Input: part model. Units: mm. Frame: model coordinates. Face numbers are marked on the shaded views. A direction names the side the tool comes from. Give positions to 0.01 mm unless a question says otherwise; leave off trailing zeros. Write each loop counter-clockwise with the first axis right and the second up, starting at its lowest first coordinate (ties: lowest second). Pieces come first, ordered by that corner, then holes. Notation, with made-up numbers: (-36, -17) -> (-12, -17) arc R19 cw to (-12, -2) -> close; hole circle Ø3 at (37.25, 26.25). An arc over 180 degrees is marked (long way). Answer as a JSON object with one key per item and string values. Group by question number.
from build123d import *

# Parameters (mm, degrees)
BOSS_EXTRUDE1_DEPTH       = 0.5
BOSS_EXTRUDE1_DEPTH_BACK  = 1
SKETCH1_R                 = 25
SKETCH17_R                = 24
SKETCH17_R_2              = 23
BOSS_EXTRUDE15_DEPTH      = 2
SKETCH2_R                 = 1
BOSS_EXTRUDE2_DEPTH       = 10
SKETCH12_W                = 23.219340148
SKETCH12_H                = 15.058436642
CUT_EXTRUDE2_DEPTH        = 5
SKETCH15_W                = 24.972946701
SKETCH15_H                = 16.75913787
SKETCH15_W_2              = 23.219340148
SKETCH15_H_2              = 15.058436642
BOSS_EXTRUDE13_DEPTH      = 5
BOSS_EXTRUDE14_DEPTH      = 0.0001
BOSS_EXTRUDE14_DEPTH_BACK = 1
SKETCH16_W                = 24.972946701
SKETCH16_H                = 16.75913787
BOSS_EXTRUDE16_DEPTH      = 8
BOSS_EXTRUDE17_DEPTH      = 1.301
BOSS_EXTRUDE18_DEPTH      = 4.5
REVOLVE1_ANGLE            = 195
REVOLVE1_OTHER_WAY_ANGLE  = 15
BOSS_EXTRUDE20_DEPTH      = 7.5
BOSS_EXTRUDE21_DEPTH      = 7.5
BOSS_EXTRUDE22_DEPTH      = 0.0001
BOSS_EXTRUDE22_DEPTH_BACK = 10.05
BOSS_EXTRUDE23_DEPTH      = 0.0001
BOSS_EXTRUDE23_DEPTH_BACK = 5.2001
REVOLVE2_ANGLE            = 90
BOSS_EXTRUDE25_DEPTH      = 12.41001
REVOLVE3_ANGLE            = 90
BOSS_EXTRUDE26_DEPTH      = 3.41001
BOSS_EXTRUDE27_DEPTH      = 0.001
BOSS_EXTRUDE27_DEPTH_BACK = 8.41001
BOSS_EXTRUDE28_DEPTH      = 7.001
BOSS_EXTRUDE29_START      = 5
SKETCH39_R                = 25
SKETCH39_R_2              = 24
SKETCH39_R_3              = 23
SKETCH39_R_4              = 22
BOSS_EXTRUDE29_DEPTH      = 5


# Read off the part's stored shape, not the designer's step: Boss-Extrude18
with BuildPart() as part:
    # Sketch1 → Boss-Extrude1 (new, two sides: drawn at the far end of the back side and taken through both)
    with BuildSketch(Plane(origin=(0, 0, 0), x_dir=(1, 0, 0), z_dir=(0, 1, 0)).offset(-BOSS_EXTRUDE1_DEPTH_BACK)):
        with Locations(Location((0, 0, 0), (0, 0, 270))):
            Circle(SKETCH1_R)
    extrude(amount=BOSS_EXTRUDE1_DEPTH + BOSS_EXTRUDE1_DEPTH_BACK)

    # Sketch17 → Boss-Extrude15 (add)
    with BuildSketch(Plane(origin=(0, 0.5, 0), x_dir=(1, 0, 0), z_dir=(0, 1, 0))):
        with Locations(Location((0, 0, 0), (0, 0, 270))):
            Circle(SKETCH17_R)
        with Locations(Location((0, 0, 0), (0, 0, 270))):
            Circle(SKETCH17_R_2, mode=Mode.SUBTRACT)
    extrude(amount=BOSS_EXTRUDE15_DEPTH)

    # Sketch2 → Boss-Extrude2 (add)
    with BuildSketch(Plane(origin=(0, 0.5, 0), x_dir=(1, 0, 0), z_dir=(0, 1, 0))):
        with Locations(Location((5, 17.917691699, 0), (0, 0, 270))):
            Circle(SKETCH2_R)
    extrude(amount=BOSS_EXTRUDE2_DEPTH)

    # Sketch12 → Cut-Extrude2 (cut)
    with BuildSketch(Plane(origin=(0, 0.5, 0), x_dir=(1, 0, 0), z_dir=(0, 1, 0))):
        with Locations((0.666876956, 9.102631979)):
            Rectangle(SKETCH12_W, SKETCH12_H)
    extrude(amount=-CUT_EXTRUDE2_DEPTH, mode=Mode.SUBTRACT)

    # Sketch15 → Boss-Extrude13 (add)
    with BuildSketch(Plane.XZ.offset(1)):
        with Locations((0.596477735, -9.107727728)):
            Rectangle(SKETCH15_W, SKETCH15_H)
        with Locations((0.666876956, -9.102631979)):
            Rectangle(SKETCH15_W_2, SKETCH15_H_2, mode=Mode.SUBTRACT)
    extrude(amount=BOSS_EXTRUDE13_DEPTH)

    # Sketch3 → Boss-Extrude16 (add)
    with BuildSketch(Plane(origin=(0, 0.5, 0), x_dir=(1, 0, 0), z_dir=(0, 1, 0))):
        Polygon((-11.97807381, -2.465798727), (-11.97807381, -1), (-21, -1), (-21, 7.575525784), (-22, 7.575525784), (-22, -2.465798727), align=None)
        with BuildLine():
            ThreePointArc((22.005108017, 8.247740366), (21.658944991, 9.118119426), (21.278371263, 9.97401205))
            Line((21.278371263, 9.97401205), (21.005108017, 9.97401205))
            Line((21.005108017, 9.97401205), (21.005108017, -1.02598795))
            Line((21.005108017, -1.02598795), (16.80718978, -1.02598795))
            Line((16.80718978, -1.02598795), (16.80718978, -2.458711062))
            Line((16.80718978, -2.458711062), (22.005108017, -2.458711062))
            Line((22.005108017, -2.458711062), (22.005108017, 8.247740366))
        make_face()
    extrude(amount=BOSS_EXTRUDE16_DEPTH)

    # Sketch18 → Boss-Extrude17 (add)
    with BuildSketch(Plane(origin=(0, 0.5, 0), x_dir=(1, 0, 0), z_dir=(0, 1, 0))):
        Polygon((0, -2.402962183), (0, -0.862974972), (-5.282158739, -0.862974972), (-5.282158739, -14.003106764), (0, -14.003106764), (0, -12.402962183), (-3.5, -12.402962183), (-3.5, -2.402962183), align=None)
        Polygon((15.094136196, -0.862974972), (0.201079682, -0.862974972), (0.559908327, -2.402962183), (13.5, -2.402962183), (13.5, -12.402962183), (2.889983811, -12.402962183), (3.262829577, -14.003106764), (15.094136196, -14.003106764), align=None)
        Polygon((2.889983811, -12.402962183), (0, -12.402962183), (0, -14.003106764), (3.262829577, -14.003106764), align=None)
        Polygon((0.201079682, -0.862974972), (0, -0.862974972), (0, -2.402962183), (0.559908327, -2.402962183), align=None)
    extrude(amount=BOSS_EXTRUDE17_DEPTH)

    # Boss-Extrude18 outline → Boss-Extrude18 (add)
    with BuildSketch(Plane(origin=(0, 0.5, 0), x_dir=(1, 0, 0), z_dir=(0, 1, 0))):
        with BuildLine():
            Line((20.724842186, 9.97401205), (18.818512993, 9.97401205))
            Line((18.818512993, 9.97401205), (18.818512993, 9.972233135))
            Line((18.818512993, 9.972233135), (16.80718978, 9.972233135))
            Line((16.80718978, 9.972233135), (16.80718978, -1.02598795))
            Line((16.80718978, -1.02598795), (18.818512993, -1.02598795))
            Line((18.818512993, -1.02598795), (18.818512993, 7.959494075))
            Line((18.818512993, 7.959494075), (21.005108017, 7.959494075))
            Line((21.005108017, 7.959494075), (21.005108017, 9.369388304))
            ThreePointArc((21.005108017, 9.369388304), (20.867165079, 9.672715314), (20.724842186, 9.97401205))
        make_face()
        Polygon((-13.988084857, -1), (-11.97807381, -1), (-11.97807381, 7.575525784), (-21, 7.575525784), (-21, 5.565099869), (-13.988084857, 5.565099869), align=None)
    extrude(amount=BOSS_EXTRUDE18_DEPTH)

    # Sketch22 → Revolve1 (revolve)
    with BuildSketch(Plane(origin=(0, 0, -17.487296663), x_dir=(-1, 0, 0), z_dir=(0, 0, -1))):
        Polygon((-4.976750106, 2.5), (-4.976750106, 4.97103297), (-5.944220353, 4.97103297), (-7.362854562, -1), (-4.976750106, -1), align=None)
    revolve(axis=Axis((4.976750106, 2.5, -17.487296663), (0, 1, 0)), revolution_arc=REVOLVE1_ANGLE)

    # Sketch22 → Revolve1 other way (revolve)
    with BuildSketch(Plane(origin=(0, 0, -17.487296663), x_dir=(-1, 0, 0), z_dir=(0, 0, -1))):
        Polygon((-4.976750106, 2.5), (-4.976750106, 4.97103297), (-5.944220353, 4.97103297), (-7.362854562, -1), (-4.976750106, -1), align=None)
    revolve(axis=Axis((4.976750106, 2.5, -17.487296663), (0, -1, 0)), revolution_arc=REVOLVE1_OTHER_WAY_ANGLE)

    # Sketch23 → Boss-Extrude20 (add)
    with BuildSketch(Plane(origin=(0, 0, 1), x_dir=(-1, 0, 0), z_dir=(0, 0, -1))):
        Polygon((21, 0.5), (21, 2.00493968), (19.5, 0.5), align=None)
    extrude(amount=BOSS_EXTRUDE20_DEPTH)

    # Sketch24 → Boss-Extrude21 (add)
    with BuildSketch(Plane.ZY.offset(13.988084857)):
        Polygon((1, 0.5), (1, 2), (-0.5, 0.5), align=None)
    extrude(amount=BOSS_EXTRUDE21_DEPTH)

    # Sketch25 → Boss-Extrude22 (add, two sides: drawn at the far end of the back side and taken through both)
    with BuildSketch(Plane(origin=(-11.97807381, 0, 0), x_dir=(0, 0, -1), z_dir=(1, 0, 0)).offset(-BOSS_EXTRUDE22_DEPTH_BACK)):
        Polygon((-2.465798727, 0.5), (-3.965798727, 0.5), (-2.465798727, 2), align=None)
    extrude(amount=BOSS_EXTRUDE22_DEPTH + BOSS_EXTRUDE22_DEPTH_BACK)

    # Sketch28 → Boss-Extrude23 (add, two sides: drawn at the far end of the back side and taken through both)
    with BuildSketch(Plane.ZY.offset(-16.80718978).offset(-BOSS_EXTRUDE23_DEPTH_BACK)):
        Polygon((2.458711062, 2.003228909), (2.458711062, 0.5), (3.95259513, 0.5), align=None)
    extrude(amount=BOSS_EXTRUDE23_DEPTH + BOSS_EXTRUDE23_DEPTH_BACK)

    # Sketch30 → Revolve2 (revolve)
    with BuildSketch(Plane.ZY.offset(-16.80708978)):
        Polygon((2.458711062, 2.003228909), (2.458711062, 0.5), (3.95259513, 0.5), align=None)
    revolve(axis=Axis((16.80708978, 2.003228909, 2.458711062), (0, -1, 0)), revolution_arc=REVOLVE2_ANGLE)

    # Sketch31 → Boss-Extrude25 (add)
    with BuildSketch(Plane(origin=(0, 0, 2.458711062), x_dir=(-1, 0, 0), z_dir=(0, 0, -1))):
        Polygon((-16.792249437, 1.988295734), (-16.792249437, 0.5), (-15.313205712, 0.5), align=None)
    extrude(amount=BOSS_EXTRUDE25_DEPTH)

    # Sketch32 → Revolve3 (revolve)
    with BuildSketch(Plane(origin=(0, 0, -9.951298938), x_dir=(-1, 0, 0), z_dir=(0, 0, -1))):
        Polygon((-16.792249437, 1.988295734), (-16.792249437, 0.5), (-15.313205712, 0.5), align=None)
    revolve(axis=Axis((16.792249437, 1.988295734, -9.951298938), (0, -1, 0)), revolution_arc=REVOLVE3_ANGLE)

    # Sketch33 → Boss-Extrude26 (add)
    with BuildSketch(Plane(origin=(16.792249437, 0, 0), x_dir=(0, 0, -1), z_dir=(1, 0, 0))):
        Polygon((9.951298938, 1.988295734), (11.430342663, 0.5), (9.951298938, 0.5), (9.915470666, 0.5), (9.915470666, 1.988295734), align=None)
    extrude(amount=BOSS_EXTRUDE26_DEPTH)

    # Sketch34 → Boss-Extrude27 (add, two sides: drawn at the far end of the back side and taken through both)
    with BuildSketch(Plane(origin=(-11.97807381, 0, 0), x_dir=(0, 0, -1), z_dir=(1, 0, 0)).offset(-BOSS_EXTRUDE27_DEPTH_BACK)):
        Polygon((7.575525784, 0.5), (9.075525784, 0.5), (7.575525784, 2), align=None)
    extrude(amount=BOSS_EXTRUDE27_DEPTH + BOSS_EXTRUDE27_DEPTH_BACK)

    # Sketch37 → Boss-Extrude28 (add)
    with BuildSketch(Plane.XY.offset(-5.565099869)):
        Polygon((-13.988084857, 0.5), (-13.988084857, 2), (-15.488084857, 0.5), align=None)
    extrude(amount=BOSS_EXTRUDE28_DEPTH)


with BuildPart() as body_2:
    # Sketch16 → Boss-Extrude14 (new, two sides: drawn at the far end of the back side and taken through both)
    with BuildSketch(Plane(origin=(0, -6, 0), x_dir=(-1, 0, 0), z_dir=(0, -1, 0)).offset(-BOSS_EXTRUDE14_DEPTH_BACK)):
        with Locations((-0.596477735, 9.107727728)):
            Rectangle(SKETCH16_W, SKETCH16_H)
    extrude(amount=BOSS_EXTRUDE14_DEPTH + BOSS_EXTRUDE14_DEPTH_BACK)


    add(part.part)  # Boss-Extrude29 merges part
    # Sketch39 → Boss-Extrude29 (add)
    # profile 1 of 2: a face of its own
    with BuildSketch(Plane.XZ.offset(1).offset(BOSS_EXTRUDE29_START)):
        with Locations(Location((0, 0, 0), (0, 0, 90))):
            Circle(SKETCH39_R)
        with Locations(Location((0, 0, 0), (0, 0, 90))):
            Circle(SKETCH39_R_2, mode=Mode.SUBTRACT)
    # profile 2 of 2: a face of its own
    with BuildSketch(Plane.XZ.offset(1).offset(BOSS_EXTRUDE29_START)):
        with Locations(Location((0, 0, 0), (0, 0, 90))):
            Circle(SKETCH39_R_3)
        with Locations(Location((0, 0, 0), (0, 0, 270))):
            Circle(SKETCH39_R_4, mode=Mode.SUBTRACT)
    extrude(amount=-BOSS_EXTRUDE29_DEPTH)


solid = body_2.part
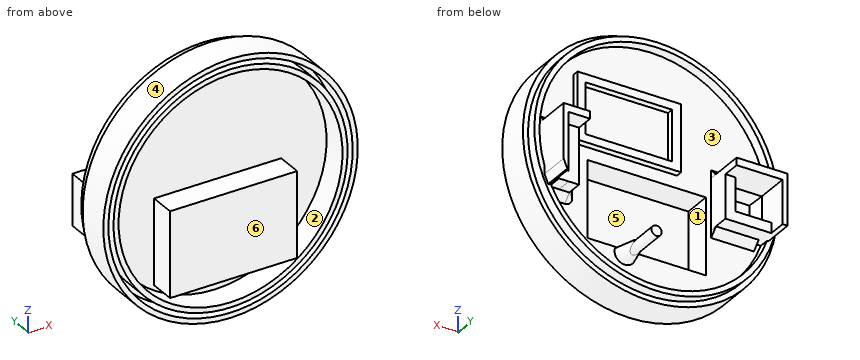
1. Section A-A (y = -1.75). Return the cut outline in (x, z).
2. Mould query, pull axis X, two halves, no side actions, for the marked faces 3, 4, 5 and 6. Classes: pulls with the +X half, pulls with the -X half, needs draft (parallel to the pull), parting line crosses it, or undercut.
3. Line query: line 1 (X direction, y = -3.65, z = 0); line 2 (Z direction, x = 20.5, y = 3); line 3 (X direction, y = 7.25, z = -6.5). Output: solid intervals per line, ascending.
4. Contact query for flat-ended pins moving along their axis: pin 1 Ø1.5 at (y, z) = (2.5, 3.5) entering from +X; pin 2 Ø4 at (x, z) = (20.5, -5.5) entering from +Y; pin 3 Ø1.4 at (y, z) = (1, 9.5) entering from +X. Output: stop coordinate, or through.
5. Section B-B (y = 5.75). Return the cut outline in (x, z), plus the area to 3 significant figures.
6. Reachability of the marked faces 1 and 2 from +Z, -Z, +X, -X, +Y, -Y: full face, straight path, thin tool, end or side. Return the list, or none.
Working result:
{
 "1": {"outline": "circle Ø50 at (0, 0); circle Ø46 at (0, 0); (-11.89, -17.49) -> (13.08, -17.49) -> (13.08, -0.73) -> (-11.89, -0.73) -> close; hole circle Ø48 at (0, 0); hole circle Ø44 at (0, 0); hole (-10.94, -16.63) -> (12.28, -16.63) -> (12.28, -1.57) -> (-10.94, -1.57) -> close"},
 "2": {"face 3": "undercut", "face 4": "parting line crosses it", "face 5": "undercut", "face 6": "needs draft"},
 "3": {"line 1": "x = -25 to -24, -23 to -22, 22 to 23, 24 to 25", "line 2": "z = -9.97 to -7.96, 1.03 to 2.46", "line 3": "x = -22 to -21, 21.01 to 22.01"},
 "4": {"pin 1": "stops at x = 23.84", "pin 2": "stops at y = 8.5", "pin 3": "stops at x = 23.32"},
 "5": {"outline": "(-22, -7.58) -> (-21, -7.58) -> (-21, 1) -> (-11.98, 1) -> (-11.98, 2.47) -> (-22, 2.47) -> close; circle Ø2 at (5, -17.92); (16.81, 1.03) -> (21.01, 1.03) -> (21.01, -9.97) -> (21.28, -9.97) arc R23.5 ccw to (22.01, -8.25) -> (22.01, 2.46) -> (16.81, 2.46) -> close", "area": "44.3 mm^2"},
 "6": {"face 1": "+Y", "face 2": "-Y"}
}
